from build123d import *

# Parameters (mm, degrees)
SKETCH1_W              = 300
SKETCH1_H              = 50
BASE_FLANGE1_DEPTH     = 3.175
SKETCHED_BEND2_DEPTH   = 50
SKETCHED_BEND2_2_DEPTH = 50
SKETCH7_R              = 4.815
CUT_EXTRUDE1_DEPTH     = 10
SKETCH8_R              = 1.5
SKETCH8_R_2            = 0.75
CUT_EXTRUDE2_DEPTH     = 10
CUT_EXTRUDE3_DEPTH     = 140.094007146


# Read off the part's stored shape, not the designer's step: Sketched Bend2
# Sheet-metal steps are written as plain solids
with BuildPart() as part:
    # Sketch1 → Base-Flange1 (new body)
    with BuildSketch(Plane(origin=(0, 0, 0), x_dir=(1, 0, 0), z_dir=(0, 1, 0))):
        with Locations((0, -25)):
            Rectangle(SKETCH1_W, SKETCH1_H)
    extrude(amount=-BASE_FLANGE1_DEPTH)

    # Sketched Bend2 outline → Sketched Bend2 (cut)
    with BuildSketch(Plane.XY):
        with BuildLine():
            Line((-150, -3.175), (-34.919, -3.175))
            ThreePointArc((-34.919, -3.175), (-37.164417556, -2.245124663), (-38.094999843, 0))
            Line((-38.094999843, 0), (-150, 0))
            Line((-150, 0), (-150, -3.175))
        make_face()
        with BuildLine():
            ThreePointArc((38.094999843, 0), (37.164417556, -2.245124663), (34.919, -3.175))
            Line((34.919, -3.175), (150, -3.175))
            Line((150, -3.175), (150, 0))
            Line((150, 0), (38.094999843, 0))
        make_face()
    extrude(amount=SKETCHED_BEND2_DEPTH, mode=Mode.SUBTRACT)

    # Sketched Bend2 2 outline → Sketched Bend2 2 (add)
    with BuildSketch(Plane.XY):
        with BuildLine():
            ThreePointArc((-38.095, 0.001), (-38.094999961, 0.0005), (-38.094999843, 0))
            Line((-38.094999843, 0), (-34.919, 0))
            ThreePointArc((-34.919, 0), (-34.919707107, 0.000292893), (-34.92, 0.001))
            Line((-34.92, 0.001), (-34.92, 105.082))
            Line((-34.92, 105.082), (-38.095, 105.082))
            Line((-38.095, 105.082), (-38.095, 0.001))
        make_face()
        with BuildLine():
            Line((34.919, 0), (38.094999843, 0))
            ThreePointArc((38.094999843, 0), (38.094999961, 0.0005), (38.095, 0.001))
            Line((38.095, 0.001), (38.095, 105.082))
            Line((38.095, 105.082), (34.92, 105.082))
            Line((34.92, 105.082), (34.92, 0.001))
            ThreePointArc((34.92, 0.001), (34.919707107, 0.000292893), (34.919, 0))
        make_face()
    extrude(amount=SKETCHED_BEND2_2_DEPTH)

    # Sketch7 → Cut-Extrude1 (cut)
    with BuildSketch(Plane(origin=(38.095, 0, 0), x_dir=(0, 0, -1), z_dir=(1, 0, 0))):
        with Locations(Location((-25, 80.082, 0), (0, 0, 90))):
            Circle(SKETCH7_R)
    extrude(amount=-CUT_EXTRUDE1_DEPTH, mode=Mode.SUBTRACT)

    # Sketch8 → Cut-Extrude2 (cut)
    with BuildSketch(Plane.ZY.offset(38.095)):
        with Locations(Location((25, 80.082, 0), (0, 0, 270))):
            Circle(SKETCH8_R)
        with Locations(Location((25, 87.582, 0), (0, 0, 270))):
            Circle(SKETCH8_R_2)
        with Locations(Location((25, 72.582, 0), (0, 0, 270))):
            Circle(SKETCH8_R_2)
    extrude(amount=-CUT_EXTRUDE2_DEPTH, mode=Mode.SUBTRACT)

    # Sketch9 → Cut-Extrude3 (cut, through all)
    with BuildSketch(Plane.ZY.offset(38.095)):
        with BuildLine():
            Line((0, 105.082), (0, 80.082))
            ThreePointArc((0, 80.082), (7.32233047, 97.75966953), (25, 105.082))
            Line((25, 105.082), (0, 105.082))
        make_face()
        with BuildLine():
            ThreePointArc((25, 105.082), (42.67766953, 97.75966953), (50, 80.082))
            Line((50, 80.082), (50, 105.082))
            Line((50, 105.082), (25, 105.082))
        make_face()
    extrude(amount=-CUT_EXTRUDE3_DEPTH, mode=Mode.SUBTRACT)


solid = part.part
Verification items for the finished model (mm, model axes). A direction names the side the tool comes from. Coordinates: 2 decimals unless noted, no trailing zeros. Loops run counter-clockwise (first coordinate to the right, second up) from the corner with the lowest first, then second, coordinate; pieces in that order, holes last. Notation, with made-up numbers: M 42.5,1.25 L 73.5,1.25 A30 ccw 73.5,31.25 Z; hole C 42.25,16 d3. An arc over 180 degrees is marked long. One line per item, written item: value.
1. Section check A-A on y = 20.5. Record the cut outline in (x, z) (3 decimals), plus the area to 4 significant figures.
Answers follow:
outline: M -38.095,0 L -34.92,0 L -34.92,50 L -38.095,50 Z; M 34.92,0 L 38.095,0 L 38.095,50 L 34.92,50 Z
area: 317.5 mm^2
2. Gauge pin test, flat ends, axial feed: P1, Ø11, axis at y = 80.082, z = 25, coming from the +X side (3 decimals); P2, Ø1.5, axis at x = 24, z = 27.5, coming from the +Y side; P3, Ø2.5, axis at y = 80.082, z = 25, coming from the -X side; P4, Ø0.9, axis at y = 87.582, z = 25, coming from the -X side. Record the tip position at first contact, or that the pin passes through.
Answers follow:
P1: x = 38.095
P2: y = 0
P3: through
P4: x = 34.92
3. Material ranges on line 1 along X through (y, z) = (39, 32) (3 decimals); line 2 along Y through (x, z) = (30, 35) (3 decimals), recorded low to high. Write a range as from..to.
Answers follow:
line 1: -38.095..-34.92, 34.92..38.095
line 2: -3.175..0
4. Set-up check for faces 1 (the flat face through (0, 0, 25)), 2 (the flat face through (0, -1, 0)): record each of +Z, -Z, +X, -X, +Y, -Y from which the full face is reachable in a straight line by a thin tool's end or side.
Answers follow:
face 1: +Z, -Z, +Y
face 2: -Z, +X, -X, +Y, -Y
5. Mould release check, pull along Y, two halves, no side actions. Record for faces 3 (the cylindrical face through (-36.53, 81.58, 25.07)), 4 (the flat face through (34.92, 53, 25)), 5 (the cylindrical face through (36.53, 84.53, 23.16)), 6 (the cylindrical face through (37.19, -2.22, 24.65)): pulls with the +Y half, pulls with the -Y half, needs draft (parallel to the pull), parting line crosses it, or undercut.
Answers follow:
face 3: undercut
face 4: needs draft
face 5: undercut
face 6: pulls with the -Y half
6. Section check C-C on x = 6. Record the cut outline in (y, z) (3 decimals), plus the area to 3 significant figures.
Answers follow:
outline: M -3.175,0 L 0,0 L 0,50 L -3.175,50 Z
area: 159 mm^2
